Geometry check sheet. Reference: the model listing, model coordinates, mm. A direction names the side the tool comes from. Round coordinates to 2 decimals unless told otherwise and drop trailing zeros. Order: outer loops, then holes, each group sorted by start corner. A loop starts at its lowest first (then second) coordinate and runs counter-clockwise, first axis right, second up. Notation, with made-up numbers: (35, 11.25) - (52, 11.25) arc R22 cw to (52, 20.25) - close; hole circle Ø10 at (34.25, -26). An arc over 180 degrees is marked (long way). One line per question, with ' | ' between items. Start each with the question number.
Q1. Gauge pin test, flat ends, axial feed: P1, Ø1.5, axis at y = 1, z = -12.5, coming from the -X side; P2, Ø3, axis at x = -7, z = -1, coming from the +Y side; P3, Ø2.5, axis at y = 4, z = -7, coming from the +X side. Record the tip position at first contact, or that the pin passes through.
Q2. Material ranges on line 1 along Z through (x, y) = (-8, 4.75); line 2 along Z through (x, y) = (-8, 0.2), recorded low to high.
Q3. Sectioned sample at D-D, the plane z = 0. Give the number of separate pieces and of enclosed holes in the cut face, then the cut area to 3 significant figures.
Q4. Sectioned sample at A-A, the plane z = -8. Enter the section's corners in (x, y), then the cut area to 3 significant figures.
Q5. Tool access check on faces 4 (the face through (-13.09, 7.41, -0.92)), 5 (the face through (-10.398, 3.943, -8.106)), 6 (the face through (-11.7, 4, -10)), 7 (the face through (-10, 0.8, -2)), 8 (the face through (-4.3, 4, -10)). Record the directions out of +Z, -Z, +X, -X, +Y, -Y that give a thin tool (end or side, any length) a straight path to the whole face; none if there is none.
Q6. Sectioned sample at B-B, the plane x = -17.75. Enter the section's corners in (y, z).
Q7. Sectioned sample at C-C, the plane y = 6. Enter the section's corners in (x, z).
Q8. Mould release check, pull along X, two halves, no side actions. Record for faces 1 (the face through (-19.7, 3.8, -0.1)), 2 (the face through (-10.25, 7.41, -18.06)), 3 (the face through (-8.1, 7.8, -4.6)): +X half, -X half, draft (parallel to the pull), parting line (faces both ways), or undercut.
```python
from build123d import *

# Parameters (mm, degrees)
BOSS_EXTRUDE3_DEPTH = 7.8
SKETCH2_R           = 2.4
CUT_EXTRUDE1_DEPTH  = 7.8
SKETCH3_R           = 3.05
CUT_EXTRUDE2_DEPTH  = 0.8
SKETCH4_R           = 3.05
SKETCH4_R_2         = 3.129900969
CUT_EXTRUDE3_DEPTH  = 0.8


with BuildPart() as part:
    # Sketch1 → Boss-Extrude3 (new body)
    with BuildSketch(Plane(origin=(0, 0, 0), x_dir=(1, 0, 0), z_dir=(0, 1, 0))):
        with BuildLine():
            Line((-16, -3.7), (0, -3.7))
            ThreePointArc((0, -3.7), (3.7, 0), (0, 3.7))
            Line((0, 3.7), (-4.3, 3.7))
            Line((-4.3, 3.7), (-4.3, 16))
            ThreePointArc((-4.3, 16), (-8, 19.7), (-11.7, 16))
            Line((-11.7, 16), (-11.7, 3.7))
            Line((-11.7, 3.7), (-16, 3.7))
            ThreePointArc((-16, 3.7), (-19.7, 0), (-16, -3.7))
        make_face()
    extrude(amount=BOSS_EXTRUDE3_DEPTH)

    # Sketch2 → Cut-Extrude1 (cut)
    with BuildSketch(Plane(origin=(0, 7.8, 0), x_dir=(1, 0, 0), z_dir=(0, 1, 0))):
        Circle(SKETCH2_R)
        with Locations((-16, 0)):
            Circle(SKETCH2_R)
        with Locations((-8, 0)):
            Circle(SKETCH2_R)
        with Locations((-8, 8)):
            Circle(SKETCH2_R)
        with Locations((-8, 16)):
            Circle(SKETCH2_R)
    extrude(amount=-CUT_EXTRUDE1_DEPTH, mode=Mode.SUBTRACT)

    # Sketch3 → Cut-Extrude2 (cut)
    with BuildSketch(Plane(origin=(0, 7.8, 0), x_dir=(1, 0, 0), z_dir=(0, 1, 0))):
        Circle(SKETCH3_R)
        with Locations((-16, 0)):
            Circle(SKETCH3_R)
        with Locations((-8, 0)):
            Circle(SKETCH3_R)
        with Locations((-8, 8)):
            Circle(SKETCH3_R)
        with Locations((-8, 16)):
            Circle(SKETCH3_R)
    extrude(amount=-CUT_EXTRUDE2_DEPTH, mode=Mode.SUBTRACT)

    # Sketch4 → Cut-Extrude3 (cut)
    with BuildSketch(Plane.XZ):
        Circle(SKETCH4_R)
        with Locations((-16, 0)):
            Circle(SKETCH4_R)
        with Locations((-8, 0)):
            Circle(SKETCH4_R)
        with Locations((-8, -16)):
            Circle(SKETCH4_R_2)
        with Locations((-8, -8)):
            Circle(SKETCH4_R)
    extrude(amount=-CUT_EXTRUDE3_DEPTH, mode=Mode.SUBTRACT)


solid = part.part
```
Determined:
1) P1: stops at x = -11.7 | P2: stops at y = 7 | P3: stops at x = -4.3
2) line 1: z = -19.7 to -18.4, -13.6 to -10.4, -5.6 to -2.4, 2.4 to 3.7 | line 2: z = -19.7 to -19.13, -12.87 to -11.05, -4.95 to -3.05, 3.05 to 3.7
3) separate pieces: 4 | enclosed holes: 0 | area: 64.0 mm2
4) outline: (-11.7, 0) - (-11.05, 0) - (-11.05, 0.8) - (-10.4, 0.8) - (-10.4, 7) - (-11.05, 7) - (-11.05, 7.8) - (-11.7, 7.8) - close; (-5.6, 0.8) - (-4.95, 0.8) - (-4.95, 0) - (-4.3, 0) - (-4.3, 7.8) - (-4.95, 7.8) - (-4.95, 7) - (-5.6, 7) - close | area: 18.2 mm2
5) face 4: +Y | face 5: +Y, -Y | face 6: -Z, -X, +Y, -Y | face 7: -Y | face 8: -Z, +X, +Y, -Y
6) outline: (0, -3.26) - (7.8, -3.26) - (7.8, -2.5) - (7, -2.5) - (7, -1.64) - (0.8, -1.64) - (0.8, -2.5) - (0, -2.5) - close; (0, 2.5) - (0.8, 2.5) - (0.8, 1.64) - (7, 1.64) - (7, 2.5) - (7.8, 2.5) - (7.8, 3.26) - (0, 3.26) - close
7) outline: (-16, -3.7) - (-11.7, -3.7) - (-11.7, -16) arc R3.7 ccw to (-4.3, -16) - (-4.3, -3.7) - (0, -3.7) arc R3.7 ccw to (0, 3.7) - (-16, 3.7) arc R3.7 ccw to start; hole circle Ø4.8 at (-16, 0); hole circle Ø4.8 at (-8, -16); hole circle Ø4.8 at (-8, -8); hole circle Ø4.8 at (-8, 0); hole circle Ø4.8 at (0, 0)
8) face 1: -X half | face 2: undercut | face 3: draft
